The model under review builds one solid part; all positions refer to its coordinate system, in mm. A direction names the side the tool comes from. Coordinates: 2 decimals unless noted, no trailing zeros. Order: outer loops, then holes, each group sorted by start corner. A loop starts at its lowest first (then second) coordinate and runs counter-clockwise, first axis right, second up. Notation, with made-up numbers: M -9,71 L 27,71 A12 cw 27,89 Z; hole C 10.25,26.25 d2. An arc over 180 degrees is marked long. One line per item, written item: value.
```python
from build123d import *

# Parameters (mm, degrees)
RESSALTO_EXTRUS_O1_DEPTH      = 16.0875
RESSALTO_EXTRUS_O1_DEPTH_BACK = 0.158383869
ESBO_O2_W                     = 6.720883869
ESBO_O2_H                     = 25
CORTE_EXTRUS_O1_DEPTH         = 55.655025447
ESBO_O3_R                     = 3.225
CORTE_EXTRUS_O2_DEPTH         = 53.127659578


with BuildPart() as part:
    # Esboço1 → Ressalto-extrusão1 (new, two sides: drawn at the far end of the back side and taken through both)
    with BuildSketch(Plane.XY.offset(-RESSALTO_EXTRUS_O1_DEPTH_BACK)):
        with BuildLine():
            ThreePointArc((-5, 12.759375), (0, 17.759375), (5, 12.759375))
            Line((5, 12.759375), (5, -12.759375))
            Line((5, -12.759375), (-5, -12.759375))
            Line((-5, -12.759375), (-5, 12.759375))
        make_face()
        Polygon((-5, -42.759375), (-5, -12.759375), (5, -12.759375), (5, 12.759375), (25, -42.759375), align=None)
    extrude(amount=RESSALTO_EXTRUS_O1_DEPTH + RESSALTO_EXTRUS_O1_DEPTH_BACK)

    # Esboço2 → Corte-extrusão1 (cut, through all)
    with BuildSketch(Plane.ZY.offset(5)):
        with Locations((7.964558066, 5.259375)):
            Rectangle(ESBO_O2_W, ESBO_O2_H)
    extrude(amount=-CORTE_EXTRUS_O1_DEPTH, mode=Mode.SUBTRACT)

    # Esboço3 → Corte-extrusão2 (cut, through all)
    with BuildSketch(Plane(origin=(0, 0, -0.158383869), x_dir=(-1, 0, 0), z_dir=(0, 0, -1))):
        with Locations((0, 12.759375)):
            Circle(ESBO_O3_R)
    extrude(amount=-CORTE_EXTRUS_O2_DEPTH, mode=Mode.SUBTRACT)


solid = part.part
```
(1) Tool access review of faces 1 (the flat face through (2, 2, 11.325)), 2 (the flat face through (-5, -15, 8)): name each direction out of +Z, -Z, +X, -X, +Y, -Y from which nothing blocks a thin tool from reaching the whole face with its end or side.
Geometry results:
face 1: +X, -X, +Y
face 2: +Z, -Z, -X, +Y, -Y
(2) We need section B-B, the plane y = -4. State the section outline as (x, z) points (1 decimal).
Geometry results:
outline: M -5,-0.2 L 11,-0.2 L 11,4.6 L -5,4.6 Z; M -5,11.3 L 11,11.3 L 11,16.1 L -5,16.1 Z
(3) For L1, parallel to Z at x = 5, y = -4 (1 decimal); L2, parallel to Y at x = 0, z = 12.4; L3, parallel to X at y = -18, z = 4.25, list the stretches that pass through material, from the lowest coordinate up.
Geometry results:
L1: z = -0.2 to 4.6, 11.3 to 16.1
L2: y = -42.76 to 9.53, 15.98 to 17.76
L3: x = -5 to 16.08
(4) Mouldability with a two-part tool opening along Z and no side actions: class faces 3 (the flat face through (2, 2, 4.604)), 4 (the flat face through (7, -19, -0.158)), 5 (the cylindrical face through (-0.11, 17.76, 13.67)), 6 (the flat face through (7, -19, 16.087)) as +Z half, -Z half, draft (parallel to the pull), parting line (faces both ways), or undercut.
Geometry results:
face 3: undercut
face 4: -Z half
face 5: draft
face 6: +Z half
(5) We need section A-A, the plane x = 0. State the section outline as (y, z) points (1 decimal), plus the area to 3 significant figures.
Geometry results:
outline: M -42.8,-0.2 L 9.5,-0.2 L 9.5,4.6 L -7.2,4.6 L -7.2,11.3 L 9.5,11.3 L 9.5,16.1 L -42.8,16.1 Z; M 16,-0.2 L 17.8,-0.2 L 17.8,4.6 L 16,4.6 Z; M 16,11.3 L 17.8,11.3 L 17.8,16.1 L 16,16.1 Z
area: 754 mm2
(6) Insertion check: pin 1 Ø6 at (y, z) = (2, 11.5) entering from +X; pin 2 Ø2 at (y, z) = (6, 10.5) entering from +X; pin 3 Ø4 at (x, z) = (9, 7.5) entering from +Y. Each pin has a flat end and moves straight along its axis. Give the tip position at first contact, or say it passes through.
Geometry results:
pin 1: stops at x = 9.96
pin 2: stops at x = 7.64
pin 3: stops at y = -7.24
(7) We need section C-C, the plane z = 13.5. State the section outline as (x, y) points (3 decimals).
Geometry results:
outline: M -5,-42.759 L 25,-42.759 L 5,12.759 A5 ccw -5,12.759 Z; hole C 0,12.759 d6.45
(8) We need section D-D, the plane x = 15. State the section outline as (y, z) points.
Geometry results:
outline: M -42.76,-0.16 L -15,-0.16 L -15,16.09 L -42.76,16.09 Z
